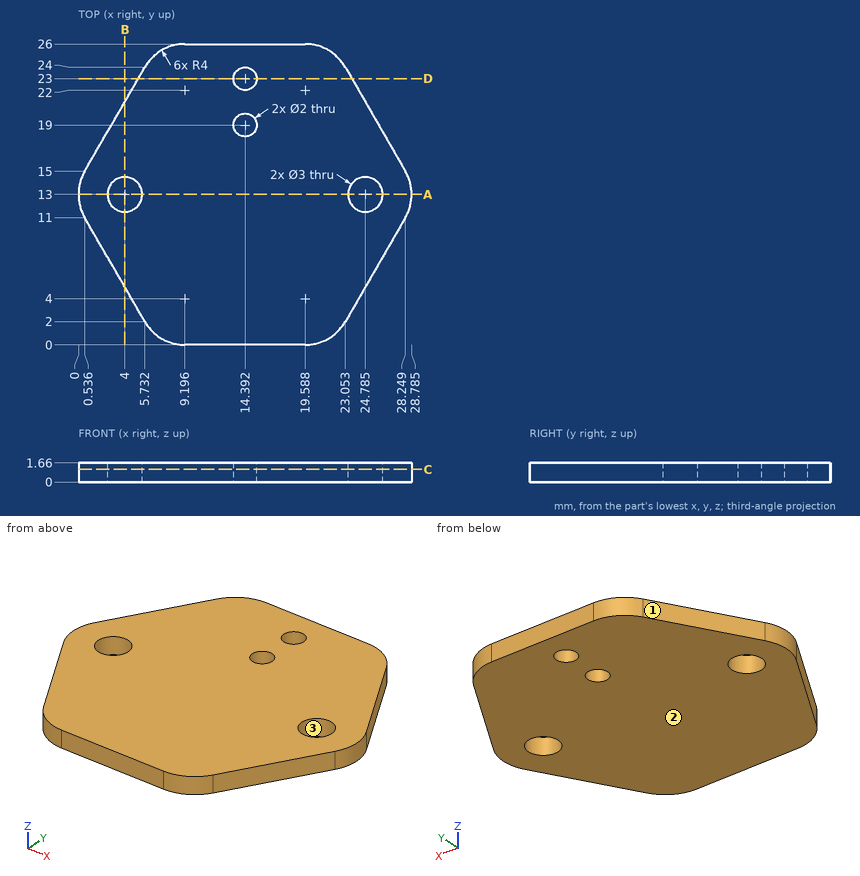
Design review of the part shown in the three views and the two pictorial views. Dimensions are in mm from the part's minimum x, y and z. Round coordinates to 2 decimals unless told otherwise and drop trailing zeros. Order: outer loops, then holes, each group sorted by start corner. A loop starts at its lowest first (then second) coordinate and runs counter-clockwise, first axis right, second up.
Q1. Wall thickness on line 1 (X direction, y = 11.75, z = 0.55) (1 decimal); line 2 (X direction, y = 2.75, z = 0.4) (1 decimal); line 3 (Y direction, x = 27, z = 0.35) (1 decimal): over which ranges is each line inside the solid? List them lowest first.
Findings below:
line 1: x = 0.2 to 3.2, 4.8 to 24, 25.6 to 28.6
line 2: x = 5.3 to 23.5
line 3: y = 8.8 to 17.2
Q2. We need section A-A, the plane y = 13. Give the boundary of the cut face in (x, z) (1 decimal).
Findings below:
outline: (0, 0) - (2.5, 0) - (2.5, 1.7) - (0, 1.7) - close; (5.5, 0) - (23.3, 0) - (23.3, 1.7) - (5.5, 1.7) - close; (26.3, 0) - (28.8, 0) - (28.8, 1.7) - (26.3, 1.7) - close
Q3. We need section D-D, the plane y = 23. Give the boundary of the cut face in (x, z) (1 decimal).
Findings below:
outline: (5.2, 0) - (13.4, 0) - (13.4, 1.7) - (5.2, 1.7) - close; (15.4, 0) - (23.6, 0) - (23.6, 1.7) - (15.4, 1.7) - close
Q4. Mouldability with a two-part tool opening along X and no side actions: class the marked faces 1, 2 and 3 as pulls with the +X half, pulls with the -X half, needs draft (parallel to the pull), parting line crosses it, or undercut.
Findings below:
face 1: pulls with the -X half
face 2: needs draft
face 3: undercut
Q5. We need section B-B, the plane x = 4. Give the boundary of the cut face in (y, z), plus the area to 3 significant figures.
Findings below:
outline: (5, 0) - (11.5, 0) - (11.5, 1.66) - (5, 1.66) - close; (14.5, 0) - (21, 0) - (21, 1.66) - (14.5, 1.66) - close
area: 21.6 mm2
Q6. Insertion check: P1, Ø4, axis at x = 4, y = 13, coming from the +Z side; P2, Ø2.5, axis at x = 24.78, y = 13, coming from the +Z side. Each pin has a flat end and moves straight along its axis. Give the tip position at first contact, or say it passes through.
Findings below:
P1: stops at z = 1.66
P2: passes through
Q7. We need section C-C, the plane z = 1.1. Give the boundary of the cut face in (x, y) (1 decimal), plus the area to 3 significant figures.
Findings below:
outline: (0.5, 11) - (5.7, 2) arc R4 ccw to (9.2, 0) - (19.6, 0) arc R4 ccw to (23.1, 2) - (28.2, 11) arc R4 ccw to (28.2, 15) - (23.1, 24) arc R4 ccw to (19.6, 26) - (9.2, 26) arc R4 ccw to (5.7, 24) - (0.5, 15) arc R4 ccw to start; hole circle Ø3 at (4, 13); hole circle Ø2 at (14.4, 19); hole circle Ø2 at (14.4, 23); hole circle Ø3 at (24.8, 13)
area: 560 mm2
